from build123d import *

# Parameters (mm, degrees)
F1_DEPTH = 18


# Not quite as in the source:
# - a feature names something its author has since deleted; it is built from what else it names


with BuildPart() as f1:
    # F0 (on Front) → F1 (new body)
    with BuildSketch(Plane.XZ):
        Polygon((0, 1000), (0, 0), (77, 0), (77, 125), (59, 125), (59, 250), (77, 250), (77, 375), (59, 375), (59, 500), (77, 500), (77, 625), (59, 625), (59, 750), (77, 750), (77, 875), (59, 875), (59, 1000), align=None)
    extrude(amount=F1_DEPTH)


solid = f1.part
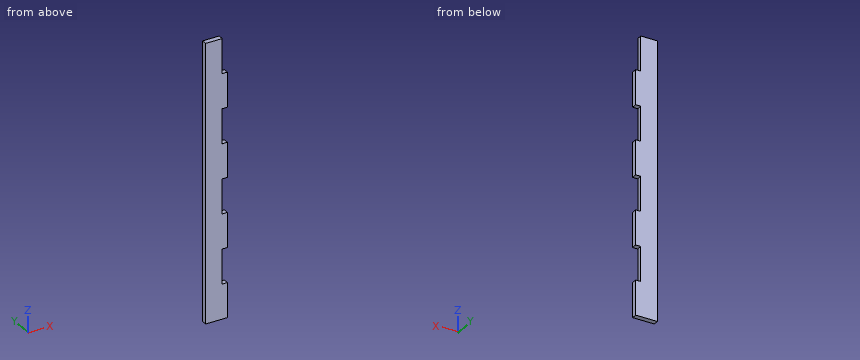
Geometry check sheet. Reference: the model listing, model coordinates, mm. Coordinates: 2 decimals unless noted, no trailing zeros. Loops run counter-clockwise (first coordinate to the right, second up) from the corner with the lowest first, then second, coordinate; pieces in that order, holes last. Notation, with made-up numbers: (69, -40) - (128, -40) arc R21 ccw to (128, -8) - close; hole circle Ø3 at (43.5, 71.25). An arc over 180 degrees is marked (long way). Use one line per item in the form item = value. Start each with the question number.
Item 1: Gauge pin test, flat ends, axial feed: pin 1 (5.5 mm diameter, centred on x = 68.5, y = -9.5, fed in from +Z); pin 2 (9 mm diameter, centred on y = -12.5, z = 947.5, fed in from +X). Record the tip position at first contact, or that the pin passes through.
Item 2: Thickness scan on probe 1 along Z at (x, y) = (71, -10.75); probe 2 along X at (y, z) = (-11.75, 648). Record the ranges inside material, lowest first.
Item 3: Section check A-A, the plane x = 68.5. Enter the section's corners in (y, z), and give its area (3 significant figures).
Item 4: Section check C-C, the plane z = 216. Enter the section's corners in (x, y).
Item 5: Section check B-B, the plane y = -5.5. Enter the section's corners in (x, z).
Computed:
q1.pin_1 = 875
q1.pin_2 = 59
q2.probe_1 = 0 to 125, 250 to 375, 500 to 625, 750 to 875
q2.probe_2 = 0 to 59
q3.outline = (-18, 0) - (0, 0) - (0, 125) - (-18, 125) - close; (-18, 250) - (0, 250) - (0, 375) - (-18, 375) - close; (-18, 500) - (0, 500) - (0, 625) - (-18, 625) - close; (-18, 750) - (0, 750) - (0, 875) - (-18, 875) - close
q3.area = 9,000 mm2
q4.outline = (0, -18) - (59, -18) - (59, 0) - (0, 0) - close
q5.outline = (0, 0) - (77, 0) - (77, 125) - (59, 125) - (59, 250) - (77, 250) - (77, 375) - (59, 375) - (59, 500) - (77, 500) - (77, 625) - (59, 625) - (59, 750) - (77, 750) - (77, 875) - (59, 875) - (59, 1000) - (0, 1000) - close
